Geometry check sheet. Reference: drawing and pictorial views, mm from the part's lowest x, y, z. A direction names the side the tool comes from. Round coordinates to 2 decimals unless told otherwise and drop trailing zeros. Loops run counter-clockwise (first coordinate to the right, second up) from the corner with the lowest first, then second, coordinate; pieces in that order, holes last. Notation, with made-up numbers: (-1, 51) - (48, 51) arc R9 cw to (48, 55) - close; hole circle Ø11 at (-36, 48). An arc over 180 degrees is marked (long way). Return JSON: item names as keys, results as strings.
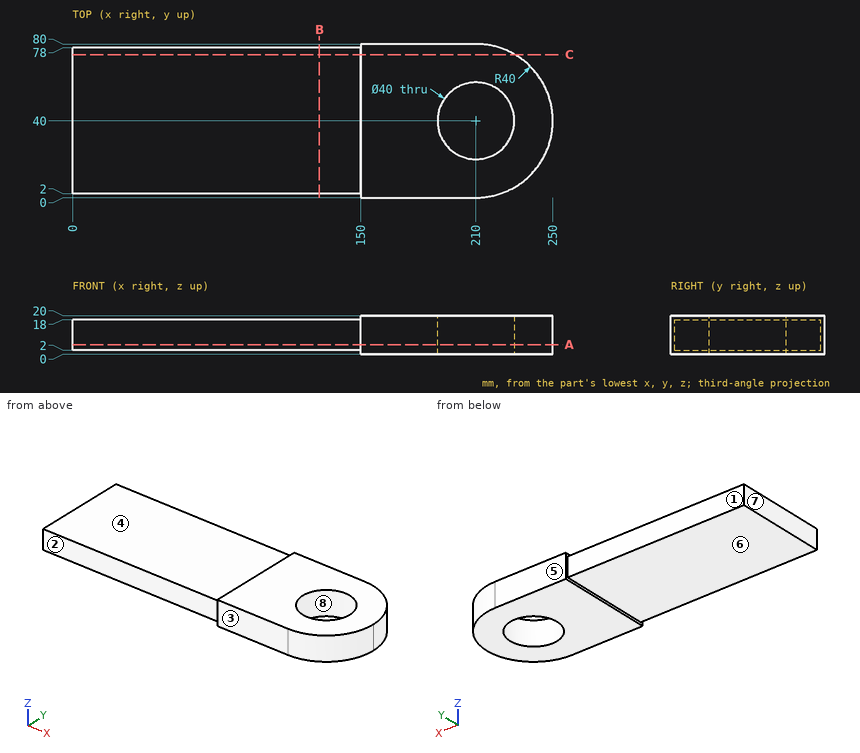
Q1. Depth check by flat-ended pin: P1, Ø1.5, axis at x = 47, z = 14.5, coming from the -Y side; P2, Ø10, axis at y = 9, z = 10.5, coming from the +X side; P3, Ø8, axis at y = 17, z = 4.5, coming from the +X side. Enter the tip coordinate at first touch or a pass-through.
Answer key:
{"P1": "stops at y = 2", "P2": "stops at x = 240.4", "P3": "stops at x = 245.2"}
Q2. Sectioned sample at B-B (x = 128.5). Enter the section's corners in (y, z).
Answer key:
{"outline": "(2, 2) - (78, 2) - (78, 18) - (2, 18) - close"}
Q3. Sectioned sample at A-A (z = 5). Enter the section's corners in (x, y).
Answer key:
{"outline": "(0, 2) - (150, 2) - (150, 0) - (210, 0) arc R40 ccw to (210, 80) - (150, 80) - (150, 78) - (0, 78) - close; hole circle Ø40 at (210, 40)"}
Q4. Tool access check on the marked faces 1, 2, 3, 4 and 5. Record the directions out of +Z, -Z, +X, -X, +Y, -Y that give a thin tool (end or side, any length) a straight path to the whole face; none if there is none.
Answer key:
{"face 1": "+Z, -Z, -X, +Y", "face 2": "+Z, -Z, -X, -Y", "face 3": "+Z, -Z, +X, -X, -Y", "face 4": "+Z, -X, +Y, -Y", "face 5": "+Z, -Z, +X, -X, +Y"}
Q5. Scan lines: probe 1 along Y at (x, z) = (210, 11); probe 2 along Z at (x, y) = (87, 20.5); probe 3 along X at (y, z) = (46, 1.25). Record each from-to range of solid material in increasing order. Write a range as [from, to].
Answer key:
{"probe 1": "y = [0, 20], [60, 80]", "probe 2": "z = [2, 18]", "probe 3": "x = [150, 190.92], [229.08, 249.55]"}
Q6. Draft check along X on the marked faces 6, 7 and 8. Enter one of: released by +X, released by -X, zero draft, split by the parting line, or undercut.
Answer key:
{"face 6": "zero draft", "face 7": "released by -X", "face 8": "undercut"}
Q7. Sectioned sample at C-C (y = 74.5). Enter the section's corners in (x, z), plus the area to 3 significant figures.
Answer key:
{"outline": "(0, 2) - (150, 2) - (150, 0) - (230.24, 0) - (230.24, 20) - (150, 20) - (150, 18) - (0, 18) - close", "area": "4,000 mm²"}
